Design review of the part built by this model. Coordinates are the model's own, in mm. Face numbers are marked on the shaded views. Coordinates: 2 decimals unless noted, no trailing zeros. Write each loop counter-clockwise with the first axis right and the second up, starting at its lowest first coordinate (ties: lowest second). Pieces come first, ordered by that corner, then holes. Notation, with made-up numbers: M 85.5,-6.5 L 136.5,-6.5 A14 ccw 136.5,9.5 Z; hole C 19,-20.75 d5. An arc over 180 degrees is marked long. Return JSON: item names as keys, results as strings. Group by question number.
```python
from build123d import *

# Parameters (mm, degrees)
SKETCH1_R           = 2.5527
BOSS_EXTRUDE1_DEPTH = 3.175
FILLET1_R           = 4.7625


with BuildPart() as part:
    # Sketch1 → Boss-Extrude1 (new body)
    with BuildSketch(Plane.XY):
        Polygon((-27.051, 31.75), (-27.051, -29.21), (34.925, -29.21), (34.925, -7.62), (-10.795, -7.62), (-10.795, 31.75), align=None)
        with Locations((-19.05, -19.05)):
            Circle(SKETCH1_R, mode=Mode.SUBTRACT)
        with Locations((-19.05, -6.35)):
            Circle(SKETCH1_R, mode=Mode.SUBTRACT)
        with Locations((12.7, -19.05)):
            Circle(SKETCH1_R, mode=Mode.SUBTRACT)
        with Locations((25.4, -19.05)):
            Circle(SKETCH1_R, mode=Mode.SUBTRACT)
        with Locations((-19.05, 6.35)):
            Circle(SKETCH1_R, mode=Mode.SUBTRACT)
        with Locations((-19.05, 19.05)):
            Circle(SKETCH1_R, mode=Mode.SUBTRACT)
        with Locations((-19.05, -19.05)):
            Circle(SKETCH1_R)
    extrude(amount=BOSS_EXTRUDE1_DEPTH)

    # Fillet1
    fillet1_edges = [part.edges().sort_by_distance(p)[0] for p in [
        (-27.051, 31.75, 1.5875),
        (-10.795, 31.75, 1.5875),
        (-10.795, -7.62, 1.5875),
        (34.925, -7.62, 1.5875),
        (34.925, -29.21, 1.5875),
        (-27.051, -29.21, 1.5875),
    ]]
    fillet(fillet1_edges, radius=FILLET1_R)

    # Sketch2 → CSK for #10 Flat Head Machine Screw1 (revolve, cut)
    with BuildSketch(Plane(origin=(0, -19.05, 3.175), x_dir=(0, -1, 0), z_dir=(1, 0, 0))):
        Polygon((0, 0), (0, 3.175), (2.5527, 3.175), (2.5527, 2.688180894), (4.8895, 0), align=None)
    revolve(axis=Axis((0, -19.05, 9.525), (0, 0, -1)), mode=Mode.SUBTRACT)


solid = part.part
```
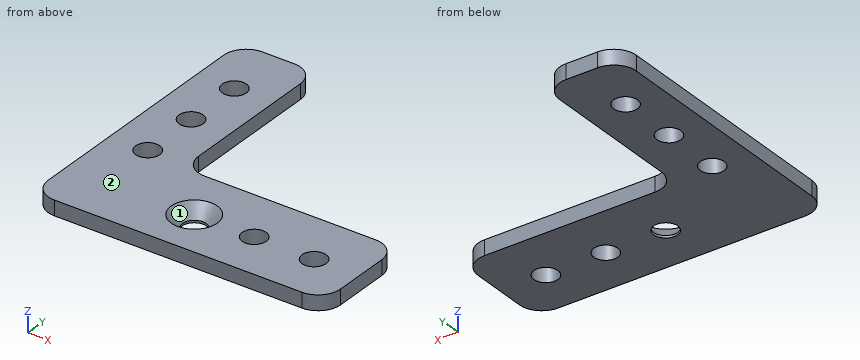
Item 1: Add section A-A (y = -19.05). Write out the cut boundary in (x, z) (1 decimal), plus the area to 3 significant figures.
Item 2: Add section B-B (x = 12.7). Write out the cut boundary in (y, z) (3 decimals).
Item 3: For pin 1 (3 mm diameter, centred on x = -1, y = -21.5, fed in from +Z); pin 2 (4 mm diameter, centred on x = 12.7, y = -19.05, fed in from -Z); pin 3 (1 mm diameter, centred on y = 14.5, z = 2, fed in from +X) (3 decimals); pin 4 (1.6 mm diameter, centred on x = 3, z = 1.5, fed in from +Y), all flat-tipped, find the tip position at first contact; note any pin that passes through.
Item 4: The part is to be moulded in two halves that separate along X. For the marked faces 1 and 2, say which applies: pulls with the +X half, pulls with the -X half, needs draft (parallel to the pull), parting line crosses it, or undercut.
Item 5: Add section D-D (x = 0). Write out the cut boundary in (y, z) (1 decimal).
Item 6: Add section C-C (y = 4.5). Write out the cut boundary in (x, z) (3 decimals).
Item 7: For line 1 (Y direction, x = -19.05, z = 0.7); line 2 (Y direction, x = 7.5, z = 2.55); line 3 (X direction, y = -17.5, z = 1.85) (3 decimals), list the stretches that pass through material, from the lowest coordinate up.
Geometry check:
{
 "1": {"outline": "M -27.1,0 L -2.6,0 L -2.6,0.5 L -4.9,3.2 L -27.1,3.2 Z; M 2.6,0 L 10.1,0 L 10.1,3.2 L 4.9,3.2 L 2.6,0.5 Z; M 15.3,0 L 22.8,0 L 22.8,3.2 L 15.3,3.2 Z; M 28,0 L 34.9,0 L 34.9,3.2 L 28,3.2 Z", "area": "142 mm^2"},
 "2": {"outline": "M -29.21,0 L -21.603,0 L -21.603,3.175 L -29.21,3.175 Z; M -16.497,0 L -7.62,0 L -7.62,3.175 L -16.497,3.175 Z"},
 "3": {"pin 1": "z = 2.32", "pin 2": "through", "pin 3": "x = -10.795", "pin 4": "y = -7.62"},
 "4": {"face 1": "undercut", "face 2": "needs draft"},
 "5": {"outline": "M -29.2,0 L -21.6,0 L -21.6,0.5 L -23.9,3.2 L -29.2,3.2 Z; M -16.5,0 L -7.6,0 L -7.6,3.2 L -14.2,3.2 L -16.5,0.5 Z"},
 "6": {"outline": "M -27.051,0 L -20.809,0 L -20.809,3.175 L -27.051,3.175 Z; M -17.291,0 L -10.795,0 L -10.795,3.175 L -17.291,3.175 Z"},
 "7": {"line 1": "-29.21 to -8.9, -3.8 to 3.8, 8.9 to 16.5, 21.6 to 31.75", "line 2": "-29.21 to -7.62", "line 3": "-27.051 to -3.401, 3.401 to 10.672, 14.728 to 23.372, 27.428 to 34.925"}
}
